For this review, take the finished solid that the model builds, in its own axes (mm). A direction names the side the tool comes from. Round coordinates to 2 decimals unless told otherwise and drop trailing zeros. Order: outer loops, then holes, each group sorted by start corner. A loop starts at its lowest first (then second) coordinate and runs counter-clockwise, first axis right, second up. Notation, with made-up numbers: (27, 57.25) - (78, 57.25) arc R35 cw to (78, 96.25) - close; hole circle Ø9 at (37, 29.25). An arc over 180 degrees is marked (long way). One line per item, written item: value.
```python
from build123d import *

# Parameters (mm, degrees)
EXTRUDE_1_DEPTH     = 48
SKETCH_2_W          = 48
SKETCH_2_H          = 48
EXTRUDE_2_DEPTH     = 48
SKETCH_3_W          = 40
SKETCH_3_H          = 40
CUT_EXTRUDE_1_DEPTH = 84
SKETCH_4_W          = 40
SKETCH_4_H          = 40
CUT_EXTRUDE_2_DEPTH = 84
SKETCH_5_W          = 40
SKETCH_5_H          = 40
CUT_EXTRUDE_3_DEPTH = 84
SKETCH_6_W          = 48
SKETCH_6_H          = 48
EXTRUDE_5_DEPTH     = 44


with BuildPart() as part:
    # 草图1 → 凸台-拉伸1 (new body)
    with BuildSketch(Plane(origin=(0, 0, 0), x_dir=(1, 0, 0), z_dir=(0, 1, 0))):
        Polygon((0, 88), (0, 0), (88, 0), (88, 48), (48, 48), (48, 88), align=None)
    extrude(amount=EXTRUDE_1_DEPTH)

    # 草图2 → 凸台-拉伸2 (add)
    with BuildSketch(Plane(origin=(0, 48, 0), x_dir=(1, 0, 0), z_dir=(0, 1, 0))):
        with Locations((24, 24)):
            Rectangle(SKETCH_2_W, SKETCH_2_H)
    extrude(amount=EXTRUDE_2_DEPTH)

    # 草图3 → 切除-拉伸1 (cut)
    with BuildSketch(Plane(origin=(88, 0, 0), x_dir=(0, 0, -1), z_dir=(1, 0, 0))):
        with Locations((24, 24)):
            Rectangle(SKETCH_3_W, SKETCH_3_H)
    extrude(amount=-CUT_EXTRUDE_1_DEPTH, mode=Mode.SUBTRACT)

    # 草图4 → 切除-拉伸2 (cut)
    with BuildSketch(Plane(origin=(0, 0, -88), x_dir=(-1, 0, 0), z_dir=(0, 0, -1))):
        with Locations((-24, 24)):
            Rectangle(SKETCH_4_W, SKETCH_4_H)
    extrude(amount=-CUT_EXTRUDE_2_DEPTH, mode=Mode.SUBTRACT)

    # 草图5 → 切除-拉伸3 (cut)
    with BuildSketch(Plane(origin=(0, 96, 0), x_dir=(1, 0, 0), z_dir=(0, 1, 0))):
        with Locations((24, 24)):
            Rectangle(SKETCH_5_W, SKETCH_5_H)
    extrude(amount=-CUT_EXTRUDE_3_DEPTH, mode=Mode.SUBTRACT)

    # 草图6 → 凸台-拉伸5 (add)
    with BuildSketch(Plane(origin=(4, 0, 0), x_dir=(0, 0, -1), z_dir=(1, 0, 0))):
        with Locations((24, 24)):
            Rectangle(SKETCH_6_W, SKETCH_6_H)
    extrude(amount=EXTRUDE_5_DEPTH)


solid = part.part
```
Item 1: The part is to be moulded in two halves that separate along X. For faces 6 (the flat face through (4, 24, -68)), 7 (the flat face through (0, 37, -34)), 8 (the flat face through (24, 48, -68)), say which applies: +X half, -X half, draft (parallel to the pull), parting line (faces both ways), or undercut.
Returned:
face 6: undercut
face 7: -X half
face 8: draft
Item 2: Machinability: for faces 1 (the flat face through (68, 4, -24)), 2 (the flat face through (68, 24, -48)), 3 (the flat face through (4, 72, -24)), 4 (the flat face through (24, 44, -68)), 5 (the flat face through (48, 72, -24)), which of the approach directions +Z, -Z, +X, -X, +Y, -Y give a long, thin tool a straight path to every point of the face, cutting with its end or side? Answer none if there is none.
Returned:
face 1: +X
face 2: -Z, +X, +Y, -Y
face 3: +Y
face 4: -Z
face 5: +Z, -Z, +X, +Y
Item 3: Take a section at D-D (x = 11.5). Write out the cut boundary in (y, z).
Returned:
outline: (0, -88) - (4, -88) - (4, -48) - (44, -48) - (44, -88) - (48, -88) - (48, -48) - (96, -48) - (96, -44) - (48, -44) - (48, -4) - (96, -4) - (96, 0) - (0, 0) - close
Item 4: Wall thickness on line 1 (Y direction, x = 80, z = -26); line 2 (Z direction, x = 14.5, y = 85): over which ranges is each line inside the solid? List them lowest first.
Returned:
line 1: 0 to 4, 44 to 48
line 2: -48 to -44, -4 to 0
Item 5: Take a section at A-A (y = 73). Write out the cut boundary in (x, z).
Returned:
outline: (0, -48) - (48, -48) - (48, 0) - (0, 0) - close; hole (4, -44) - (44, -44) - (44, -4) - (4, -4) - close
Item 6: For P1, Ø3, axis at x = 77.5, z = -13, coming from the +Y side; P2, Ø12, axis at x = 32, y = 70, coming from the -Z side; P3, Ø20, axis at y = 21, z = -32, coming from the +X side, all flat-tipped, find the tip position at first contact; note any pin that passes through.
Returned:
P1: y = 48
P2: z = -48
P3: x = 48
Item 7: Take a section at C-C (y = 9). Write out the cut boundary in (x, z).
Returned:
outline: (0, -88) - (4, -88) - (4, -48) - (44, -48) - (44, -88) - (48, -88) - (48, -48) - (88, -48) - (88, -44) - (48, -44) - (48, -4) - (88, -4) - (88, 0) - (0, 0) - close
